```python
from build123d import *

# Parameters (mm, degrees)
BOSS_EXTRUDE1_DEPTH              = 50.8
CUT_EXTRUDE1_DEPTH               = 47.8
BOSS_EXTRUDE2_DEPTH              = 3
SKETCH4_W                        = 44.8
SKETCH4_H                        = 47.8
CUT_EXTRUDE2_DEPTH               = 3
SKETCH5_W                        = 44.8
SKETCH5_H                        = 47.8
CUT_EXTRUDE3_DEPTH               = 3
SKETCH6_W                        = 10
SKETCH6_H                        = 10
SKETCH6_H_2                      = 20
BOSS_EXTRUDE3_DEPTH              = 3
FILLET1_R                        = 5
FILLET2_R                        = 3
M3_5_CLEARANCE_HOLE2_D           = 3.9
M3_5_CLEARANCE_HOLE2_CSINK_D     = 3.95
M3_5_CLEARANCE_HOLE2_CSINK_ANGLE = 90


with BuildPart() as part:
    # Sketch1 → Boss-Extrude1 (new body)
    with BuildSketch(Plane(origin=(0, 0, 0), x_dir=(1, 0, 0), z_dir=(0, 1, 0))):
        with BuildLine():
            Line((0, 0), (0, 50.8))
            Line((0, 50.8), (-50.8, 50.8))
            ThreePointArc((-50.8, 50.8), (0, 101.6), (50.8, 50.8))
            Line((50.8, 50.8), (50.8, 0))
            Line((50.8, 0), (0, 0))
        make_face()
    extrude(amount=BOSS_EXTRUDE1_DEPTH)

    # Sketch2 → Cut-Extrude1 (cut)
    with BuildSketch(Plane(origin=(0, 50.8, 0), x_dir=(1, 0, 0), z_dir=(0, 1, 0))):
        with BuildLine():
            Line((3, 3), (47.8, 3))
            Line((47.8, 3), (47.8, 50.8))
            ThreePointArc((47.8, 50.8), (1.500739839, 98.576435404), (-47.705764851, 53.8))
            Line((-47.705764851, 53.8), (3, 53.8))
            Line((3, 53.8), (3, 3))
        make_face()
    extrude(amount=-CUT_EXTRUDE1_DEPTH, mode=Mode.SUBTRACT)

    # Sketch3 → Boss-Extrude2 (add)
    with BuildSketch(Plane(origin=(0, 50.8, 0), x_dir=(1, 0, 0), z_dir=(0, 1, 0))):
        with BuildLine():
            Line((0, 50.8), (0, 0))
            Line((0, 0), (50.8, 0))
            Line((50.8, 0), (50.8, 50.8))
            ThreePointArc((50.8, 50.8), (0, 101.6), (-50.8, 50.8))
            Line((-50.8, 50.8), (0, 50.8))
        make_face()
    extrude(amount=BOSS_EXTRUDE2_DEPTH)

    # Sketch4 → Cut-Extrude2 (cut)
    with BuildSketch(Plane.XY):
        with Locations((25.4, 26.9)):
            Rectangle(SKETCH4_W, SKETCH4_H)
    extrude(amount=-CUT_EXTRUDE2_DEPTH, mode=Mode.SUBTRACT)

    # Sketch5 → Cut-Extrude3 (cut)
    with BuildSketch(Plane.XY.offset(-50.8)):
        with Locations((-25.4, 26.9)):
            Rectangle(SKETCH5_W, SKETCH5_H)
    extrude(amount=-CUT_EXTRUDE3_DEPTH, mode=Mode.SUBTRACT)

    # Sketch6 → Boss-Extrude3 (add)
    with BuildSketch(Plane.XY):
        with Locations((25.4, 58.8)):
            Rectangle(SKETCH6_W, SKETCH6_H)
        with Locations((55.8, 26.9)):
            Rectangle(SKETCH6_W, SKETCH6_H_2)
        with Locations((25.4, -5)):
            Rectangle(SKETCH6_W, SKETCH6_H)
    extrude(amount=-BOSS_EXTRUDE3_DEPTH)

    # Fillet1
    fillet1_edges = [part.edges().sort_by_distance(p)[0] for p in [
        (3, 50.8, -26.9),
        (47.8, 50.8, -25.4),
        (1.500739839, 50.8, -98.576435404),
        (3, 3, -26.9),
        (1.500739839, 3, -98.576435404),
        (47.8, 3, -25.4),
        (0, 53.8, -25.4),
        (50.8, 53.8, -25.4),
        (0, 53.8, -101.6),
        (0, 0, -25.4),
        (0, 0, -101.6),
        (50.8, 0, -25.4),
    ]]
    fillet(fillet1_edges, radius=FILLET1_R)

    # Fillet2
    fillet2_edges = [part.edges().sort_by_distance(p)[0] for p in [
        (30.4, 0, -1.5),
        (30.4, -10, -1.5),
        (20.4, -10, -1.5),
        (20.4, 0, -1.5),
        (20.4, 53.8, -1.5),
        (20.4, 63.8, -1.5),
        (30.4, 63.8, -1.5),
        (30.4, 53.8, -1.5),
        (50.8, 16.9, -1.5),
        (50.8, 36.9, -1.5),
        (60.8, 36.9, -1.5),
        (60.8, 16.9, -1.5),
    ]]
    fillet(fillet2_edges, radius=FILLET2_R)

    # M3.5 Clearance Hole2 (through all)
    with Locations(Plane(origin=(0, 0, -3), x_dir=(-1, 0, 0), z_dir=(0, 0, -1))):
        with Locations((-55.8, 31.9), (-55.8, 21.9), (-25.4, 58.8), (-25.4, -5)):
            CounterSinkHole(M3_5_CLEARANCE_HOLE2_D / 2, M3_5_CLEARANCE_HOLE2_CSINK_D / 2, counter_sink_angle=M3_5_CLEARANCE_HOLE2_CSINK_ANGLE)


solid = part.part
```
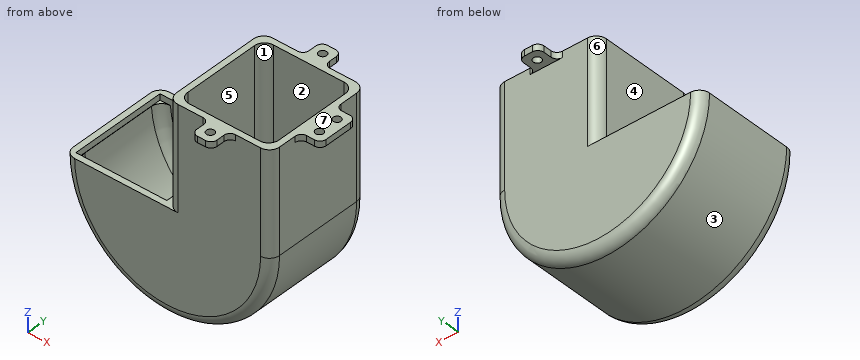
Input: part model. Units: mm. Frame: model coordinates. Face numbers are marked on the shaded views. A direction names the side the tool comes from. Give positions to 0.01 mm unless a question says otherwise; leave off trailing zeros. Write each loop counter-clockwise with the first axis right and the second up, starting at its lowest first coordinate (ties: lowest second). Pieces come first, ordered by that corner, then holes. Notation, with made-up numbers: (-34, 65.5) - (23, 65.5) arc R24 ccw to (23, 104.5) - close; hole circle Ø10 at (26.25, 73). An arc over 180 degrees is marked (long way). Write item = value, one per line. Start each with the question number.
1) Material intervals for L1, parallel to Y at x = 25.4, z = -0.6; L2, parallel to X at y = 31.9, z = -1.7; L3, parallel to Y at x = 55.8, z = -0.6, sorted ascending. Write a range as [from, to].
2) Cut plane A-A (y = 31.9). Return loops of the section in (x, z) (3 decimals), and give its area (3 significant figures).
3) Cut plane C-C (z = -29.5). Return loops of the section in (x, y), and give its area (3 significant figures).
4) Draft query along X for the marked faces 1, 2, 3 and 4. Return one class per face: pulls with the +X half, pulls with the -X half, needs draft (parallel to the pull), parting line crosses it, or undercut.
5) Cut plane D-D (x = 25.4). Give the number of separate pieces and of enclosed holes in the cut face, and give its area (3 significant figures).
6) Cut plane B-B (y = 43). Return loops of the section in (x, z), and give its area (3 significant figures).
7) Reachability of the marked faces 5, 6 and 7 from +Z, -Z, +X, -X, +Y, -Y: full face, straight path, thin tool, end or side. Return the list, or none.
8) Pin query (flat end, axial travel): pin 1 (11 mm diameter, centred on x = 28.5, y = 58.5, fed in from -Z); pin 2 (1 mm diameter, centred on y = 33.5, z = -66.5, fed in from -X); pin 3 (2 mm diameter, centred on y = 8, z = -10.5, fed in from -X); pin 4 (3 mm diameter, centred on x = 55.8, y = 31.9, fed in from +Z). Return the tip coordinate at first contact, or that it passes through.
Answers follow:
q1.L1 = [-10, -6.95], [-3.05, 3], [50.8, 56.85], [60.75, 63.8]
q1.L2 = [0, 3], [47.8, 53.85], [57.75, 60.8]
q1.L3 = [16.9, 19.95], [23.85, 29.95], [33.85, 36.9]
q2.outline = (-50.8, -50.8) arc R50.8 ccw to (50.8, -50.8) - (50.8, -3) - (53.825, -3) - (53.85, -2.975) - (53.85, 0) - (47.8, 0) - (47.8, -50.8) arc R47.8 cw to (-47.706, -53.8) - (-47.8, -53.8) - (-47.8, -50.8) - close; (-3, -53.8) - (3, -53.8) - (3, 0) - (0, 0) - (0, -50.8) - (-3, -50.8) - close; (57.75, -2.975) - (57.775, -3) - (60.8, -3) - (60.8, 0) - (57.75, 0) - close
q2.area = 806 mm^2
q3.outline = (0, 5) arc R5 ccw to (5, 0) - (45.8, 0) arc R5 ccw to (50.8, 5) - (50.8, 48.8) arc R5 ccw to (45.8, 53.8) - (5, 53.8) arc R5 ccw to (0, 48.8) - close; hole (3, 8) arc R5 ccw to (8, 3) - (42.8, 3) arc R5 ccw to (47.8, 8) - (47.8, 45.8) arc R5 ccw to (42.8, 50.8) - (8, 50.8) arc R5 ccw to (3, 45.8) - close
q3.area = 592 mm^2
q4.face_1 = undercut
q4.face_2 = undercut
q4.face_3 = parting line crosses it
q4.face_4 = pulls with the -X half
q5.separate_pieces = 3
q5.enclosed_holes = 0
q5.area = 773 mm^2
q6.outline = (-50.8, -50.8) arc R50.8 ccw to (50.8, -50.8) - (50.8, 0) - (47.8, 0) - (47.8, -50.8) arc R47.8 cw to (-47.71, -53.8) - (-47.8, -53.8) - (-47.8, -50.8) - close; (-3, -53.8) - (3, -53.8) - (3, 0) - (0, 0) - (0, -50.8) - (-3, -50.8) - close
q6.area = 787 mm^2
q7.face_5 = +Z
q7.face_6 = +Z, -X, +Y
q7.face_7 = +Z, +X, -X, +Y, -Y
q8.pin_1 = -90.68
q8.pin_2 = -48.47
q8.pin_3 = 0
q8.pin_4 = through
